The listing builds one solid part. Answer for the finished solid, in the listing's coordinates (mm). Give positions to 0.01 mm unless a question says otherwise; leave off trailing zeros. Write each loop counter-clockwise with the first axis right and the second up, starting at its lowest first coordinate (ties: lowest second). Pieces come first, ordered by that corner, then holes. Notation, with made-up numbers: (9.5, -4) - (45.5, -4) arc R26 ccw to (45.5, 27) - close; hole circle Ø11 at (-9, -15.75). An arc over 180 degrees is marked (long way). Answer as CSV lines item,"result". Start each with the question number.
(1) Straight lines are drawn through the part: probe 1 along Y at (x, z) = (5, -1); probe 2 along Y at (x, z) = (1.75, -2.25); probe 3 along X at (y, z) = (11.75, 1.15). For each, find the intervals that lie inside material, in ascending order.
(2) Find section B-B (z = -2.05). Write down the section's boundary in (x, y), then the cut area to 3 significant figures.
(3) Each of these flat-tipped pins is pushed along its axis until it touches: pin 1 Ø2 at (y, z) = (7.5, 0) entering from +X; pin 2 Ø3 at (x, z) = (-4.5, 0) entering from +Y. Where does it stop, or does it pass through?
(4) Find section A-A (x = 9). Write down the section's boundary in (y, z), then the cut area to 3 significant figures.
from build123d import *

# Parameters (mm, degrees)
SKETCH003_W  = 15
SKETCH003_H  = 3
PAD002_DEPTH = 6


with BuildPart() as obj1:
    # Sketch003 → Revolution (revolve)
    with BuildSketch(Plane.XZ):
        with Locations((7.5, 1.5)):
            Rectangle(SKETCH003_W, SKETCH003_H)
    revolve(axis=Axis((0, 0, 0), (0, 0, 1)))


with BuildPart() as part_mirroring:
    # Part__Mirroring: instance of obj1
    add(obj1.part.mirror(Plane(origin=(0, 0, 0), x_dir=(0, 1, 0), z_dir=(0, 0, 1))))


with BuildPart() as obj2:
    # Fusion001 base: copy of obj1
    add(obj1.part)

    # Fusion001: union Part__Mirroring
    add(part_mirroring.part)

    # Sketch004 → Pad002 (new body)
    with BuildSketch(Plane.XY.offset(3)):
        with BuildLine():
            Line((15, 0), (15, -15))
            Line((15, -15), (-15, -15))
            Line((-15, -15), (-15, 0))
            Line((-15, 0), (-7, 0))
            ThreePointArc((-7, 0), (0, -7), (7, 0))
            Line((7, 0), (15, 0))
        make_face()
    extrude(amount=-PAD002_DEPTH)


solid = obj2.part
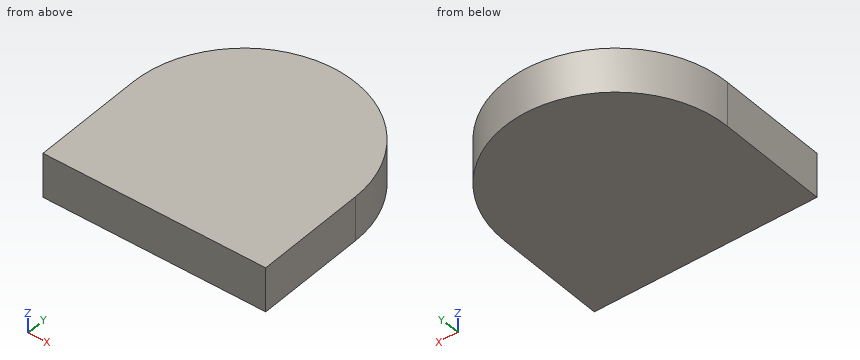
Result set:
1,probe 1,"-15 to 14.14"
1,probe 2,"-15 to 14.9"
1,probe 3,"-9.32 to 9.32"
2,outline,"(-15, -15) - (15, -15) - (15, 0) arc R15 ccw to (-15, 0) - close"
2,area,"803 mm^2"
3,pin 1,"x = 13.52"
3,pin 2,"y = 14.7"
4,outline,"(-15, -3) - (12, -3) - (12, 3) - (-15, 3) - close"
4,area,"162 mm^2"
